```python
from build123d import *

# Parameters (mm, degrees)
SKETCH1_W           = 5
SKETCH1_H           = 10
BOSS_EXTRUDE1_DEPTH = 0.6
SKETCH2_W           = 3.6
SKETCH2_H           = 10.01049857
BOSS_EXTRUDE2_DEPTH = 0.4
SKETCH4_W           = 10.01049857
SKETCH4_H           = 0.4
CUT_EXTRUDE2_DEPTH  = 0.02
SKETCH5_W           = 10.01049857
SKETCH5_H           = 0.4
CUT_EXTRUDE3_DEPTH  = 0.02


with BuildPart() as part:
    # Sketch1 → Boss-Extrude1 (new body)
    with BuildSketch(Plane(origin=(0, 0, 0), x_dir=(1, 0, 0), z_dir=(0, 1, 0))):
        with Locations((0.556994819, 3.847150259)):
            Rectangle(SKETCH1_W, SKETCH1_H)
    extrude(amount=BOSS_EXTRUDE1_DEPTH)

    # Sketch2 → Boss-Extrude2 (add)
    with BuildSketch(Plane.XZ):
        with Locations((2.756994819, -3.852399544)):
            Rectangle(SKETCH2_W, SKETCH2_H)
        with Locations((-1.643005181, -3.852399544)):
            Rectangle(SKETCH2_W, SKETCH2_H)
    extrude(amount=BOSS_EXTRUDE2_DEPTH)

    # Sketch4 → Cut-Extrude2 (cut)
    with BuildSketch(Plane(origin=(4.556994819, 0, 0), x_dir=(0, 0, -1), z_dir=(1, 0, 0))):
        with Locations((3.852399544, -0.2)):
            Rectangle(SKETCH4_W, SKETCH4_H)
    extrude(amount=-CUT_EXTRUDE2_DEPTH, mode=Mode.SUBTRACT)

    # Sketch5 → Cut-Extrude3 (cut)
    with BuildSketch(Plane.ZY.offset(3.443005181)):
        with Locations((-3.852399544, -0.2)):
            Rectangle(SKETCH5_W, SKETCH5_H)
    extrude(amount=-CUT_EXTRUDE3_DEPTH, mode=Mode.SUBTRACT)


solid = part.part
```
Can you work these out from the model? Positions are in its coordinate system, mm. Coordinates: 2 decimals unless noted, no trailing zeros. Loops run counter-clockwise (first coordinate to the right, second up) from the corner with the lowest first, then second, coordinate; pieces in that order, holes last. Notation, with made-up numbers: (-14, 29.25) -> (20, 29.25) arc R6 cw to (20, 38.25) -> close; hole circle Ø9 at (8, 27.5). An arc over 180 degrees is marked (long way). Put each result on its own line as item: value. Start each with the question number.
Q1. I want a section at C-C (x = 0.5). Write out the boundary of the cut face in (y, z), plus the area to 3 significant figures.
Q2. I want a section at A-A (y = -0.2). Write out the boundary of the cut face in (x, z).
Q3. I want a section at D-D (y = 0.25). Write out the boundary of the cut face in (x, z), plus the area to 3 significant figures.
Q4. Thinking about a two-plate mould opening in Z: for faces 1 (the face through (0.5, 0.2, 1.153)), 2 (the face through (1, 0.6, -4)), which applies, pulls with the +Z half, pulls with the -Z half, needs draft (parallel to the pull), parting line crosses it, or undercut?
Q5. I want a section at B-B (z = -8). Write out the boundary of the cut face in (x, y), plus the area to 3 significant figures.
Q6. I'm going to push a flat-ended pin straight in: P1, Ø2, axis at x = -2, z = -3.5, coming from the +Y side. Where does the tip first touch, or does it pass through?
Q7. If I drill on line 1 (X direction, y = -0.2, z = -3.75); line 2 (X direction, y = 0.1, z = -7.75); line 3 (Y direction, x = -3, z = -5), over which ranges is the centre line in solid material (lowest first)? Write a range as [from, to].
Taken from the geometry:
1. outline: (0, -8.85) -> (0.6, -8.85) -> (0.6, 1.15) -> (0, 1.15) -> close
1. area: 6.00 mm2
2. outline: (-3.42, -8.86) -> (0.16, -8.86) -> (0.16, 1.15) -> (-3.42, 1.15) -> close; (0.96, -8.86) -> (4.54, -8.86) -> (4.54, 1.15) -> (0.96, 1.15) -> close
3. outline: (-1.94, -8.85) -> (3.06, -8.85) -> (3.06, 1.15) -> (-1.94, 1.15) -> close
3. area: 50.0 mm2
4. face 1: pulls with the +Z half
4. face 2: needs draft
5. outline: (-3.42, -0.4) -> (0.16, -0.4) -> (0.16, 0) -> (0.96, 0) -> (0.96, -0.4) -> (4.54, -0.4) -> (4.54, 0) -> (3.06, 0) -> (3.06, 0.6) -> (-1.94, 0.6) -> (-1.94, 0) -> (-3.42, 0) -> close
5. area: 5.86 mm2
6. P1: stops at y = 0.6
7. line 1: x = [-3.42, 0.16], [0.96, 4.54]
7. line 2: x = [-1.94, 3.06]
7. line 3: y = [-0.4, 0]
